Verification items for the finished model (mm, model axes). Face numbers are marked on the shaded views. A direction names the side the tool comes from. Coordinates: 2 decimals unless noted, no trailing zeros. Order: outer loops, then holes, each group sorted by start corner. A loop starts at its lowest first (then second) coordinate and runs counter-clockwise, first axis right, second up. Notation, with made-up numbers: (55.25, -29) - (65.25, -29) arc R17 ccw to (65.25, -16) - close; hole circle Ø6 at (15, -6.75). An arc over 180 degrees is marked (long way). One line per question, with ' | ' between items. Start each with the question number.
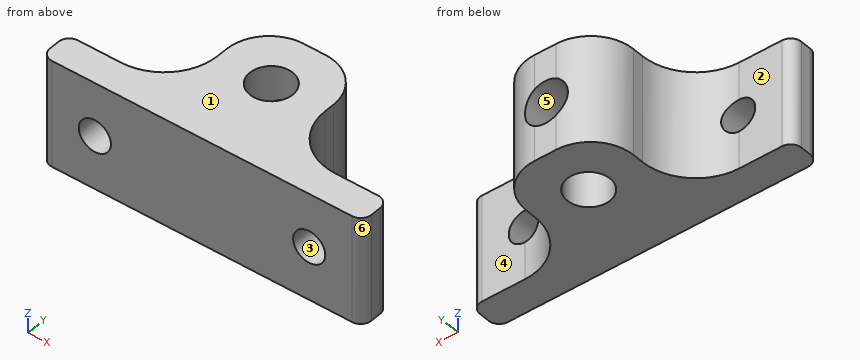
from build123d import *

# Parameters (mm, degrees)
F0_R     = 2
F1_DEPTH = 10
F2_R     = 2
F3_DEPTH = 4
F4_R     = 1.5
F5_DEPTH = 4


with BuildPart() as f1:
    # F0 (on Top) → F1 (new body)
    with BuildSketch(Plane.XY):
        with BuildLine():
            Line((-14, -1.5), (14, -1.5))
            ThreePointArc((14, -1.5), (14.707107, -1.207107), (15, -0.5))
            Line((15, -0.5), (15, 0.5))
            ThreePointArc((15, 0.5), (14.707107, 1.207107), (14, 1.5))
            Line((14, 1.5), (10, 1.5))
            ThreePointArc((10, 1.5), (6.464466, 2.964466), (5, 6.5))
            Line((5, 6.5), (5, 7.5))
            ThreePointArc((5, 7.5), (3.828427, 10.328427), (1, 11.5))
            Line((1, 11.5), (-1, 11.5))
            ThreePointArc((-1, 11.5), (-3.828427, 10.328427), (-5, 7.5))
            Line((-5, 7.5), (-5, 6.5))
            ThreePointArc((-5, 6.5), (-6.464466, 2.964466), (-10, 1.5))
            Line((-10, 1.5), (-14, 1.5))
            ThreePointArc((-14, 1.5), (-14.707107, 1.207107), (-15, 0.5))
            Line((-15, 0.5), (-15, -0.5))
            ThreePointArc((-15, -0.5), (-14.707107, -1.207107), (-14, -1.5))
        make_face()
        with Locations((0, 6.5)):
            Circle(F0_R, mode=Mode.SUBTRACT)
    extrude(amount=-F1_DEPTH)

    # F2 (on face) → F3 (cut)
    with BuildSketch(Plane(origin=(0, 11.5, 0), x_dir=(-1, 0, 0), z_dir=(0, 1, 0))):
        with Locations((0, -4.982779)):
            Circle(F2_R)
    extrude(amount=-F3_DEPTH, mode=Mode.SUBTRACT)

    # F4 (on face) → F5 (cut)
    with BuildSketch(Plane.XZ.offset(1.5)):
        with Locations((10, -5)):
            Circle(F4_R)
        with Locations((-10, -5)):
            Circle(F4_R)
    extrude(amount=-F5_DEPTH, mode=Mode.SUBTRACT)


solid = f1.part
Item 1: Section check C-C (y = 10.25). Record the cut outline in (x, z).
Item 2: Set-up check for the marked faces 4, 5 and 6: record each of +Z, -Z, +X, -X, +Y, -Y from which the full face is reachable in a straight line by a thin tool's end or side.
Item 3: Mould release check, pull along Z, two halves, no side actions. Record for the marked faces 1, 2 and 3: +Z half, -Z half, draft (parallel to the pull), parting line (faces both ways), or undercut.
Item 4: Section check A-A (z = -9.5). Record the cut outline in (x, y).
Item 5: Section check B-B (x = 0). Record the cut outline in (y, z).
Item 6: Gauge pin test, flat ends, axial feed: pin 1 (2.5 mm diameter, centred on x = 10, z = -5, fed in from +Y); pin 2 (2 mm diameter, centred on x = -12, z = -3.5, fed in from +Y); pin 3 (0.5 mm diameter, centred on y = 7, z = -3.5, fed in from -X); pin 4 (1 mm diameter, centred on x = 8, z = -8, fed in from +Y). Record the tip position at first contact, or that the pin passes through.
Item 7: Thickness scan on probe 1 along Z at (x, y) = (10, 0.95); probe 2 along Y at (x, z) = (0, -5.25); probe 3 along X at (y, z) = (7, -3.5). Record the ranges inside material, lowest first. Write a range as from..to.
Item 8: Section check D-D (x = -4). Record the cut outline in (y, z).
Completed:
1) outline: (-3.9, -10) - (3.9, -10) - (3.9, 0) - (-3.9, 0) - close; hole circle Ø4 at (0, -4.98)
2) face 4: +Z, -Z, +X, +Y | face 5: +Y | face 6: +Z, -Z, +X, -Y
3) face 1: +Z half | face 2: draft | face 3: undercut
4) outline: (-15, -0.5) arc R1 ccw to (-14, -1.5) - (14, -1.5) arc R1 ccw to (15, -0.5) - (15, 0.5) arc R1 ccw to (14, 1.5) - (10, 1.5) arc R5 cw to (5, 6.5) - (5, 7.5) arc R4 ccw to (1, 11.5) - (-1, 11.5) arc R4 ccw to (-5, 7.5) - (-5, 6.5) arc R5 cw to (-10, 1.5) - (-14, 1.5) arc R1 ccw to (-15, 0.5) - close; hole circle Ø4 at (0, 6.5)
5) outline: (-1.5, -10) - (4.5, -10) - (4.5, 0) - (-1.5, 0) - close; (8.5, -10) - (11.5, -10) - (11.5, -6.98) - (8.5, -6.98) - close; (8.5, -2.98) - (11.5, -2.98) - (11.5, 0) - (8.5, 0) - close
6) pin 1: passes through | pin 2: stops at y = 1.5 | pin 3: stops at x = -5 | pin 4: stops at y = 2.17
7) probe 1: z = -10..-6.5, -3.5..0 | probe 2: y = -1.5..4.5 | probe 3: x = -5..-1.94, 1.94..5
8) outline: (-1.5, -10) - (10.15, -10) - (10.15, 0) - (-1.5, 0) - close
